from build123d import *

# Parameters (mm, degrees)
SKETCH1_R                   = 28
BOSS_EXTRUDE1_DEPTH         = 5
FILLET1_R                   = 3
CHAMFER1_SIZE               = 1
TAP_DRILL_FOR_M3_TAP1_D     = 3
TAP_DRILL_FOR_M3_TAP1_DEPTH = 3.098709071
TAP_DRILL_FOR_M3_TAP1_TIP   = 0.901290929


with BuildPart() as part:
    # Sketch1 → Boss-Extrude1 (new body)
    with BuildSketch(Plane(origin=(0, 0, 0), x_dir=(0, 1, 0), z_dir=(0, 0, 1))):
        with Locations(Location((0, 0, 0), (0, 0, 270))):
            Circle(SKETCH1_R)
    extrude(amount=BOSS_EXTRUDE1_DEPTH)

    # Fillet1
    fillet1_edges = [part.edges().sort_by_distance(p)[0] for p in [
        (-28, 0, 5),
    ]]
    fillet(fillet1_edges, radius=FILLET1_R)

    # Sketch2 → Revolve1 (revolve)
    with BuildSketch(Plane.YZ, mode=Mode.PRIVATE) as revolve1_sk:
        Polygon((-19.075, 0), (-19.075, -2), (-20, -2), (-20, -18), (-17.5, -18), (-17.5, -8), (-12, -8), (-12, -2), (0, -2), (0, 0), align=None)
    revolve(revolve1_sk.sketch.rotate(Axis((0, 0, 0), (0, 0, 1)), 270), axis=Axis((0, 0, 0), (0, 0, 1)))

    # Chamfer1
    chamfer1_edges = [part.edges().sort_by_distance(p)[0] for p in [
        (17.5, 0, -18),
    ]]
    chamfer(chamfer1_edges, length=CHAMFER1_SIZE)

    # Tap Drill for M3 Tap1
    with Locations(Plane.XY.offset(5)):
        with Locations((0, 12.5), (-12.5, 0), (0, -12.5), (12.5, 0)):
            Hole(TAP_DRILL_FOR_M3_TAP1_D / 2, depth=TAP_DRILL_FOR_M3_TAP1_DEPTH)
            with Locations((0, 0, -(TAP_DRILL_FOR_M3_TAP1_DEPTH + TAP_DRILL_FOR_M3_TAP1_TIP / 2))):  # 118° drill point
                Cone(0, TAP_DRILL_FOR_M3_TAP1_D / 2, TAP_DRILL_FOR_M3_TAP1_TIP, mode=Mode.SUBTRACT)


solid = part.part
Read the model definition and answer for the solid it produces. Units are mm, in the model's axes. A direction names the side the tool comes from. Give positions to 0.01 mm unless a question says otherwise; leave off trailing zeros. Write each loop counter-clockwise with the first axis right and the second up, starting at its lowest first coordinate (ties: lowest second). Pieces come first, ordered by that corner, then holes. Notation, with made-up numbers: (-5.75, -33) - (39.25, -33) arc R22 cw to (39.25, -2) - close; hole circle Ø9 at (-13, 10). An arc over 180 degrees is marked (long way). Use CSV: the item, a comma, the result in double quotes. Start each with the question number.
Item 1: The part is cut by section A-A, the plane z = -10. Give the vertices of the cut face in (x, y), and give its area (3 significant figures).
Item 2: The mould has two halves that part along X. Classify faces 1 (the cylindrical face through (0, 11, 3)), 2 (the cylindrical face through (-6.07, -27.334, 0.986)), 3 (the flat face through (-6, 18, -18)): pulls with the +X half, pulls with the -X half, needs draft (parallel to the pull), parting line crosses it, or undercut.
Item 3: The part is cut by section B-B, the plane z = -5.25. Give the vertices of the cut face in (x, y).
Item 4: For faces 4 (the flat face through (18, 7, -2)), 5 (the cylindrical face through (-11.446, -3.604, -4.958)), 6 (the cylindrical face through (14, 0, 3)), determine the directions among +Z, -Z, +X, -X, +Y, -Y from which every point of the face is accessible in a straight line to the end or side of a thin tool.
Item 5: Consider line 1 (Y direction, x = 0, z = 4.3); line 2 (Z direction, x = -16, y = 11); line 3 (Y direction, x = 0, z = 2.9). Determine where each line is inside the solid, lowest interval first.
Item 6: Flat-ended cylindrical pins translate along their axes: P1, Ø21, axis at x = 0, y = 0, coming from the -Z side; P2, Ø1.5, axis at x = -16.5, y = -19, coming from the -Z side; P3, Ø5, axis at x = -5, y = -9.5, coming from the -Z side. Find the tip coordinate at first contact, or state that the pin passes through.
Taken from the geometry:
1,outline,"circle Ø40 at (0, 0); hole circle Ø35 at (0, 0)"
1,area,"295 mm2"
2,face 1,"undercut"
2,face 2,"parting line crosses it"
2,face 3,"needs draft"
3,outline,"circle Ø40 at (0, 0); hole circle Ø24 at (0, 0)"
4,face 4,"none"
4,face 5,"-Z"
4,face 6,"+Z"
5,line 1,"-26.93 to -14, -11 to 11, 14 to 26.93"
5,line 2,"-18 to -2, 0 to 5"
5,line 3,"-27.86 to -14, -11 to 11, 14 to 27.86"
6,P1,"z = -2"
6,P2,"z = 0"
6,P3,"z = -8"
